Here's how the part is built. I have some questions about the finished solid (model axes, mm). Give positions to 0.01 mm unless a question says otherwise; leave off trailing zeros. Write each loop counter-clockwise with the first axis right and the second up, starting at its lowest first coordinate (ties: lowest second). Pieces come first, ordered by that corner, then holes. Notation, with made-up numbers: (27.25, 9.25) -> (70.25, 9.25) arc R10 cw to (70.25, 20.25) -> close; hole circle Ø3 at (9, 6). An arc over 180 degrees is marked (long way). Use one line per item in the form item = value.
Autodesk Inventor part; units mm, degrees
ref_plane "YZ Plane" through (0, 0, 0) normal (1, 0, 0) x (0, 1, 0)
ref_plane "XZ Plane" through (0, 0, 0) normal (0, 1, 0) x (-1, 0, 0)
ref_plane "XY Plane" through (0, 0, 0) normal (0, 0, 1) x (1, 0, 0)
sketch "Sketch1" plane through (0, 0, 0) normal (0, 0, 1) x (1, 0, 0)
  circle A0 centre (0, 0) radius 1
  dimension "d0" = 2
extrude "Extrusion1" add sketch "Sketch1" along normal blind 3
sketch "Sketch2" plane through (0, 0, 3) normal (0, 0, 1) x (1, 0, 0)
  circle A0 centre (0, 0) radius 1
  circle A1 centre (0, 0) radius 2.55
  dimension "d3" = 5.1
extrude "Extrusion2" add sketch "Sketch2" along normal blind 5 contours A0 | A1
fillet "Fillet1" radius 0.15 1 edges at (-1, 0, 0)
sketch "Sketch3" plane through (0, 0, 0) normal (0, 0, -1) x (-1, 0, 0)
  circle A0 centre (0, 0) radius 0.85
  circle A1 centre (0, 0) radius 0.5
  dimension "d7" = 1
extrude "Extrusion3" [suppressed]
hole "Hole1" at (0, 0, 0) direction (0, 0, 1) diameter 1 depth 0.2
properties part number "Jig_Bearing_Asm_Pusher"
Q1. If I drill on line 1 along Z through (x, y) = (-0.2, -1.85); line 2 along Y through (x, z) = (0, 0.15); line 3 along X through (y, z) = (-2.3, 5), over which ranges is the centre line in solid material (lowest first)? Write a range as from..to.
Result set:
line_1 = 3..8
line_2 = -1..-0.5, 0.5..1
line_3 = -1.1..1.1
Q2. I want a section at A-A, the plane y = 0. Write out the boundary of the cut face in (x, z), and give its area (3 significant figures).
Result set:
outline = (-2.55, 3) -> (-1, 3) -> (-1, 0.15) arc R0.15 ccw to (-0.85, 0) -> (-0.5, 0) -> (-0.5, 0.2) -> (0.5, 0.2) -> (0.5, 0) -> (0.85, 0) arc R0.15 ccw to (1, 0.15) -> (1, 3) -> (2.55, 3) -> (2.55, 8) -> (-2.55, 8) -> close
area = 31.3 mm2
Q3. Will this pin go through, and if not, where does the flat tip stop? pin 1 Ø1 at (x, z) = (1, 6.5) entering from -Y.
Result set:
pin_1 = -2.5
Q4. I want a section at C-C, the plane z = 4.25. Write out the boundary of the cut face in (x, y).
Result set:
outline = circle Ø5.1 at (0, 0)
Q5. I want a section at D-D, the plane x = -1.15. Write out the boundary of the cut face in (y, z).
Result set:
outline = (-2.28, 3) -> (2.28, 3) -> (2.28, 8) -> (-2.28, 8) -> close
Q6. If we mould it in two halves opening along X, with no side actions, what happens to faces 1 (the face through (1.18, 2.26, 5.46)), 2 (the face through (0, 0, 0.2)), 3 (the face through (0, 0, 8))? For each: +X half, -X half, draft (parallel to the pull), parting line (faces both ways), or undercut.
Result set:
face_1 = parting line
face_2 = undercut
face_3 = draft
